from build123d import *

# Parameters (mm, degrees)
BOSS_EXTRUDE1_DEPTH = 6.35
SKETCH2_R           = 3
CUT_EXTRUDE3_DEPTH  = 217.426251873
BOSS_EXTRUDE3_DEPTH = 6.35
CHAMFER1_SIZE       = 8.660254038
CHAMFER1_SIZE_2     = 15
BOSS_EXTRUDE4_START = 6.35
SKETCH8_R           = 3
BOSS_EXTRUDE4_DEPTH = 6.35
SKETCH9_W           = 6.35
SKETCH9_H           = 20
BOSS_EXTRUDE5_DEPTH = 15.875
SKETCH10_R          = 3
CUT_EXTRUDE4_DEPTH  = 110.875
FILLET3_R           = 5
SKETCH11_R          = 5
CUT_EXTRUDE5_DEPTH  = 15.875


with BuildPart() as part:
    # Sketch1 → Boss-Extrude1 (new body)
    with BuildSketch(Plane(origin=(0, 0, 0), x_dir=(1, 0, 0), z_dir=(0, 1, 0))):
        Polygon((0, 0), (120, 0), (120, -50), (6.35, -173.120833333), (6.35, -180), (0, -180), align=None)
    extrude(amount=BOSS_EXTRUDE1_DEPTH)

    # Sketch2 → Cut-Extrude3 (cut, through all)
    with BuildSketch(Plane(origin=(0, 6.35, 0), x_dir=(1, 0, 0), z_dir=(0, 1, 0))):
        with Locations(Location((110, -8, 0), (0, 0, 270))):
            Circle(SKETCH2_R)
        with Locations(Location((110, -48, 0), (0, 0, 270))):
            Circle(SKETCH2_R)
        Polygon((100, -12.7), (100, -52.942838636), (12.7, -147.517838636), (12.7, -12.7), align=None)
    extrude(amount=-CUT_EXTRUDE3_DEPTH, mode=Mode.SUBTRACT)

    # Sketch7 → Boss-Extrude3 (add)
    with BuildSketch(Plane(origin=(0, 6.35, 0), x_dir=(1, 0, 0), z_dir=(0, 1, 0))):
        Polygon((116.825, -48.758626326), (4.016999063, -170.967294007), (6.35, -173.120833333), (120, -50), (120, 0), (4.016999063, 0), (4.016999063, -3.175), (116.825, -3.175), align=None)
    extrude(amount=BOSS_EXTRUDE3_DEPTH)

    # Chamfer1
    # the kernel refuses this chamfer: 15, 8.660254038 mm, written as the material it takes off along each edge
    with BuildSketch(Plane(origin=(-24.497993798, 12.7, 144.645762136), x_dir=(-0.03926825493809675, -0.9983227437537926, 0.04254060951627175), z_dir=(0.73480344462749, 0, 0.6782801027330635))) as chamfer1_piece_1_section:
        Polygon((CHAMFER1_SIZE * 0.998322743736, CHAMFER1_SIZE * 0.0578938624016), (-CHAMFER1_SIZE_2 * 0.0578938624027, CHAMFER1_SIZE_2 * 0.998322743754), (0, 0), align=None)
    chamfer1_piece_1 = extrude(amount=80.787572639, mode=Mode.PRIVATE)
    chamfer1_piece_1 = split(chamfer1_piece_1, bisect_by=Plane(origin=(8.850305535, 6.35, 168.0716905), z_dir=(0, 1, 0)), keep=Keep.TOP, mode=Mode.PRIVATE)
    add(chamfer1_piece_1, mode=Mode.SUBTRACT)
    with BuildSketch(Plane(origin=(4.016999063, 12.7, -38.80628632), x_dir=(0.9998132206222079, 0.019326765612700747, 0), z_dir=(0, 0, 1))) as chamfer1_piece_2_section:
        Polygon((CHAMFER1_SIZE_2 * 0.999813220622, -CHAMFER1_SIZE_2 * 0.0193267656127), (-CHAMFER1_SIZE * 0.0193267656124, -CHAMFER1_SIZE * 0.999813220604), (0, 0), align=None)
    chamfer1_piece_2 = extrude(amount=80.787572639, mode=Mode.PRIVATE)
    chamfer1_piece_2 = split(chamfer1_piece_2, bisect_by=Plane(origin=(9.423034105, 6.35, 1.5875), z_dir=(0, 1, 0)), keep=Keep.TOP, mode=Mode.PRIVATE)
    add(chamfer1_piece_2, mode=Mode.SUBTRACT)

    # Sketch8 → Boss-Extrude4 (add)
    # profile 1 of 2: a face of its own
    with BuildSketch(Plane(origin=(0, 6.35, 0), x_dir=(1, 0, 0), z_dir=(0, 1, 0)).offset(BOSS_EXTRUDE4_START)):
        with BuildLine():
            Line((110, -14.5), (116.825, -14.5))
            Line((116.825, -14.5), (116.825, -3.175))
            Line((116.825, -3.175), (103.5, -3.175))
            Line((103.5, -3.175), (103.5, -8))
            ThreePointArc((103.5, -8), (105.403805922, -12.596194078), (110, -14.5))
        make_face()
        with Locations(Location((110, -8, 0), (0, 0, 270))):
            Circle(SKETCH8_R, mode=Mode.SUBTRACT)
    # profile 2 of 2: a face of its own
    with BuildSketch(Plane(origin=(0, 6.35, 0), x_dir=(1, 0, 0), z_dir=(0, 1, 0)).offset(BOSS_EXTRUDE4_START)):
        with BuildLine():
            Line((110, -41.5), (116.825, -41.5))
            Line((116.825, -41.5), (116.825, -48.758626326))
            Line((116.825, -48.758626326), (103.5, -63.194042992))
            Line((103.5, -63.194042992), (103.5, -48))
            ThreePointArc((103.5, -48), (105.403805922, -43.403805922), (110, -41.5))
        make_face()
        with Locations(Location((110, -48, 0), (0, 0, 270))):
            Circle(SKETCH8_R, mode=Mode.SUBTRACT)
    extrude(amount=-BOSS_EXTRUDE4_DEPTH)

    # Sketch9 → Boss-Extrude5 (add)
    with BuildSketch(Plane(origin=(0, 6.35, 0), x_dir=(1, 0, 0), z_dir=(0, 1, 0))):
        with Locations((3.175, -10)):
            Rectangle(SKETCH9_W, SKETCH9_H)
        with Locations((3.175, -170)):
            Rectangle(SKETCH9_W, SKETCH9_H)
    extrude(amount=BOSS_EXTRUDE5_DEPTH)

    # Sketch10 → Cut-Extrude4 (cut)
    with BuildSketch(Plane(origin=(6.35, 0, 0), x_dir=(0, 0, -1), z_dir=(1, 0, 0))):
        with Locations((-10, 14.2875)):
            Circle(SKETCH10_R)
        with Locations((-170, 14.2875)):
            Circle(SKETCH10_R)
    extrude(amount=-CUT_EXTRUDE4_DEPTH, mode=Mode.SUBTRACT)

    # Fillet3
    fillet3_edges = [part.edges().sort_by_distance(p)[0] for p in [
        (103.5, 9.525, 63.194042992),
        (116.825, 9.525, 41.5),
        (116.825, 9.525, 14.5),
        (103.5, 9.525, 3.175),
        (120, 6.35, 0),
        (120, 6.35, 50),
        (6.35, 3.175, 173.120833333),
        (12.7, 3.175, 147.517838636),
        (100, 3.175, 52.942838636),
        (100, 3.175, 12.7),
        (12.7, 3.175, 12.7),
        (3.175, 22.225, 180),
        (3.175, 6.35, 160),
        (3.175, 22.225, 160),
        (3.175, 22.225, 0),
        (3.175, 22.225, 20),
        (3.175, 6.35, 20),
    ]]
    fillet(fillet3_edges, radius=FILLET3_R)

    # Sketch11 → Cut-Extrude5 (cut)
    with BuildSketch(Plane(origin=(0, 6.35, 0), x_dir=(1, 0, 0), z_dir=(0, 1, 0))):
        with Locations(Location((110, -28, 0), (0, 0, 270))):
            Circle(SKETCH11_R)
    extrude(amount=-CUT_EXTRUDE5_DEPTH, mode=Mode.SUBTRACT)


solid = part.part
For this review, take the finished solid that the model builds, in its own axes (mm). A direction names the side the tool comes from. Coordinates: 2 decimals unless noted, no trailing zeros. Write each loop counter-clockwise with the first axis right and the second up, starting at its lowest first coordinate (ties: lowest second). Pieces come first, ordered by that corner, then holes. Notation, with made-up numbers: (18, 2.5) -> (52, 2.5) arc R11 ccw to (52, 15.5) -> close; hole circle Ø2 at (81, 1). An arc over 180 degrees is marked (long way). Write each question's results on one line, items separated by ' | '. Start each with the question number.
1) The part is to be moulded in two halves that separate along X. For faces 6 (the face through (105.354, 9.569, 43.455)), 7 (the face through (118, 6, 1)), 8 (the face through (115.399, 9.481, 16.004)), say which applies: +X half, -X half, draft (parallel to the pull), parting line (faces both ways), or undercut.
2) Consider section B-B (y = 3.5). Write out the cut boundary in (x, z), plus the area to 3 significant figures.
3) For faces 1 (the face through (60.57, 3.22, 95.66)), 2 (the face through (3, 8, 180)), 3 (the face through (3, 14, 160)), 4 (the face through (53, 9, 3.175)), 5 (the face through (74, 0, 83)), list the 3-axis set-ups (+Z, -Z, +X, -X, +Y, -Y) from which the entire face can be reached by the end or side of a thin tool; tool diameter is ignored.
4) Insertion check: pin 1 (3 mm diameter, centred on y = 9, z = 28, fed in from -X) (3 decimals); pin 2 (5.5 mm diameter, centred on y = 14.29, z = 170, fed in from +X); pin 3 (3 mm diameter, centred on y = 10, z = 57, fed in from -X); pin 4 (5 mm diameter, centred on y = 6, z = 123, fed in from +X). Each pin has a flat end and moves straight along its axis. Give the tip position at first contact, or say it passes through.
5) Consider section C-C (x = 38.5). Write out the cut boundary in (y, z) (3 decimals), plus the area to 3 significant figures.
6) Consider section D-D (z = 91.5). Write out the cut boundary in (x, y).
7) Wall thickness on L1, parallel to X at y = 7.5, z = 8; L2, parallel to Y at x = 3.25, z = 10 (1 decimal); L3, parallel to Z at x = 79.5, y = 6.5 (3 decimals): over which ranges is each line inside the solid? List them lowest first. Write a range as [from, to].
8) Consider section A-A (z = 28). Write out the cut boundary in (x, y) (3 decimals), plus the area to 3 significant figures.
Geometry says:
1) face 6: -X half | face 7: +X half | face 8: undercut
2) outline: (0, 0) -> (115, 0) arc R5 ccw to (120, 5) -> (120, 48.05) arc R5 ccw to (118.67, 51.44) -> (7.68, 171.68) arc R5 cw to (6.35, 175.08) -> (6.35, 180) -> (0, 180) -> close; hole (12.7, 17.7) arc R5 ccw to (17.7, 12.7) -> (95, 12.7) arc R5 ccw to (100, 17.7) -> (100, 50.99) arc R5 ccw to (98.67, 54.38) -> (21.37, 138.12) arc R5 ccw to (12.7, 134.73) -> close; hole circle Ø10 at (110, 28); hole circle Ø6 at (110, 8); hole circle Ø6 at (110, 48) | area: 6,090 mm^2
3) face 1: +Y, -Y | face 2: +Z, +X, -X, +Y, -Y | face 3: -X, +Y | face 4: +Y | face 5: +Z, -Z, +X, -X, -Y
4) pin 1: x = 116.825 | pin 2: through | pin 3: x = 103.5 | pin 4: x = 54.92
5) outline: (0, 0) -> (12.7, 0) -> (12.7, 3.175) -> (6.35, 3.175) -> (6.35, 12.7) -> (0, 12.7) -> close; (0, 119.568) -> (6.35, 119.568) -> (6.35, 133.611) -> (12.7, 133.611) -> (12.7, 138.292) -> (0, 138.292) -> close | area: 249 mm^2
6) outline: (0, 0) -> (12.7, 0) -> (12.7, 6.35) -> (0, 6.35) -> close; (64.41, 0) -> (81.69, 0) -> (81.69, 12.7) -> (77.37, 12.7) -> (77.37, 6.35) -> (64.41, 6.35) -> close
7) L1: [0, 6.35], [103.5, 107], [113, 120] | L2: [0, 11.3], [17.3, 22.2] | L3: [0, 3.175], [89.194, 93.875]
8) outline: (0, 0) -> (12.7, 0) -> (12.7, 6.35) -> (0, 6.35) -> close; (100, 0) -> (105, 0) -> (105, 6.35) -> (100, 6.35) -> close; (115, 0) -> (120, 0) -> (120, 12.7) -> (116.825, 12.7) -> (116.825, 6.35) -> (115, 6.35) -> close | area: 164 mm^2
